```python
from build123d import *

# Parameters (mm, degrees)
SKETCH1_R           = 0.815
BOSS_EXTRUDE1_DEPTH = 0.79
SKETCH2_W           = 1.90810027
SKETCH2_H           = 0.63280283
BOSS_EXTRUDE2_DEPTH = 0.79


with BuildPart() as part:
    # Sketch1 → Boss-Extrude1 (new body)
    with BuildSketch(Plane.XY):
        with BuildLine():
            Line((-5.8, 0.599999942), (-5.8, -5.299999942))
            Line((-5.8, -5.299999942), (5.8, -5.299999942))
            Line((5.8, -5.299999942), (5.8, 0.599999942))
            ThreePointArc((5.8, 0.599999942), (5.12250756, 3.304927434), (3.249999977, 5.371166553))
            Line((3.249999977, 5.371166553), (-3.249999977, 5.371166553))
            ThreePointArc((-3.249999977, 5.371166553), (-5.12250756, 3.304927434), (-5.8, 0.599999942))
        make_face()
        with Locations(Location((0, 0.571166501, 0), (0, 0, 180))):
            Circle(SKETCH1_R, mode=Mode.SUBTRACT)
    extrude(amount=BOSS_EXTRUDE1_DEPTH)

    # Sketch2 → Boss-Extrude2 (add)
    with BuildSketch(Plane.XY.offset(0.79)):
        with Locations((0, 3)):
            Rectangle(SKETCH2_W, SKETCH2_H)
    extrude(amount=BOSS_EXTRUDE2_DEPTH)


solid = part.part
```
Here's how the part is built. I have some questions about the finished solid (model axes, mm). Give positions to 0.01 mm unless a question says otherwise; leave off trailing zeros. Order: outer loops, then holes, each group sorted by start corner. A loop starts at its lowest first (then second) coordinate and runs counter-clockwise, first axis right, second up. Notation, with made-up numbers: (11, 5.5) - (51, 5.5) arc R24 ccw to (51, 27.5) - close; hole circle Ø5 at (-21, -17.75). An arc over 180 degrees is marked (long way). Answer as a JSON object with one key per item and string values. Group by question number.
Item 1: If we section it at B-B on y = 1.25: Please give me the cut outline in (x, z), and give its area (3 significant figures).
Item 2: If we section it at A-A on x = 0: Please give me the cut outline in (y, z).
Item 3: Please list where these lines run through material, in increasing order: probe 1 along Y at (x, z) = (0, 0.5); probe 2 along Z at (x, y) = (4.25, -2.25); probe 3 along X at (y, z) = (3, 1.15).
Item 4: If we mould it in two halves opening along Y, with no side actions, what happens to faces 1 (the cylindrical face through (-5.104, 3.34, 0.389)), 2 (the cylindrical face through (-0.38, 1.29, 0.39)), 3 (the flat face through (0, -1, 0.79))? For each: pulls with the +Y half, pulls with the -Y half, needs draft (parallel to the pull), parting line crosses it, or undercut.
Item 5: If we section it at C-C on z = 0.55: Please give me the cut outline in (x, y) (3 decimals).
Item 6: If we section it at D-D on x = -2.25: Please give me the cut outline in (y, z), and give its area (3 significant figures).
Item 7: For P1, Ø0.5, axis at y = 3, z = 1.5, coming from the -X side; P2, Ø1.5, axis at x = 0, y = 0.57, coming from the +Z side; P3, Ø1.5, axis at x = -3.5, y = -2.5, coming from the +Z side; P4, Ø0.7, axis at y = 3, z = 1, coming from the +X side, each with a flat end and sliding along its axis, tell me the tip position at first contact or that it passes through.
Result set:
{
 "1": {"outline": "(-5.76, 0) - (-0.45, 0) - (-0.45, 0.79) - (-5.76, 0.79) - close; (0.45, 0) - (5.76, 0) - (5.76, 0.79) - (0.45, 0.79) - close", "area": "8.39 mm²"},
 "2": {"outline": "(-5.3, 0) - (-0.24, 0) - (-0.24, 0.79) - (-5.3, 0.79) - close; (1.39, 0) - (5.37, 0) - (5.37, 0.79) - (3.32, 0.79) - (3.32, 1.58) - (2.68, 1.58) - (2.68, 0.79) - (1.39, 0.79) - close"},
 "3": {"probe 1": "-5.3 to -0.24, 1.39 to 5.37", "probe 2": "0 to 0.79", "probe 3": "-0.95 to 0.95"},
 "4": {"face 1": "pulls with the +Y half", "face 2": "undercut", "face 3": "needs draft"},
 "5": {"outline": "(-5.8, -5.3) - (5.8, -5.3) - (5.8, 0.6) arc R5.739 ccw to (3.25, 5.371) - (-3.25, 5.371) arc R5.739 ccw to (-5.8, 0.6) - close; hole circle Ø1.63 at (0, 0.571)"},
 "6": {"outline": "(-5.3, 0) - (5.37, 0) - (5.37, 0.79) - (-5.3, 0.79) - close", "area": "8.43 mm²"},
 "7": {"P1": "x = -0.95", "P2": "through", "P3": "z = 0.79", "P4": "x = 5.39"}
}
